CAD build for the part. Positions are in the model's coordinates, mm. Face numbers are marked on the shaded views. A direction names the side the tool comes from. Give positions to 0.01 mm unless a question says otherwise; leave off trailing zeros. Write each loop counter-clockwise with the first axis right and the second up, starting at its lowest first coordinate (ties: lowest second). Pieces come first, ordered by that corner, then holes. Notation, with made-up numbers: (50, 38.5) -> (109, 38.5) arc R9 ccw to (109, 53.5) -> close; hole circle Ø2 at (12.5, 20.25). An arc over 180 degrees is marked (long way). Use one line per item in the form item = value. Start each with the question number.
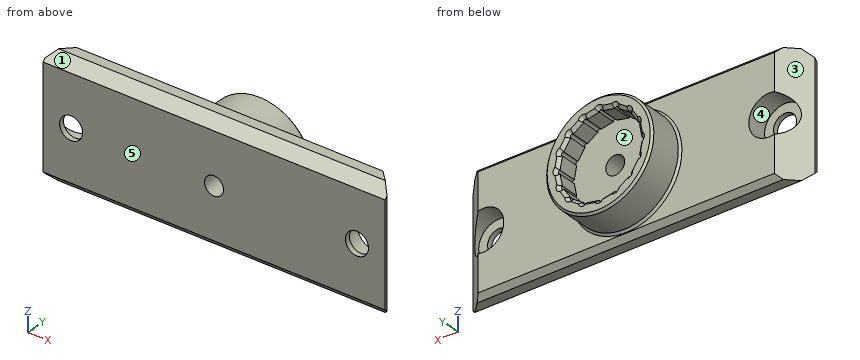
from build123d import *

# Parameters (mm, degrees)
SKETCH1_W                      = 67
SKETCH1_H                      = 24
BOSS_EXTRUDE1_DEPTH            = 5
SKETCH2_R                      = 10.5
BOSS_EXTRUDE2_DEPTH            = 7
CBORE_START                    = 1
CBORE_FOR_M4_SHCS1_OUTLINE_R   = 4
CBORE_FOR_M4_SHCS1_DEPTH       = 4
CBORE_FOR_M4_SHCS1_2_OUTLINE_R = 2.25
CBORE_FOR_M4_SHCS1_2_DEPTH     = 1
CHAMFER1_SIZE                  = 1
CHAMFER2_SIZE                  = 2
SKETCH5_OUTSIDE_W              = 83.434
SKETCH5_OUTSIDE_H              = 28.434
CUT_EXTRUDE1_DEPTH             = 43.921439864
SKETCH6_R                      = 10.5
BOSS_EXTRUDE3_DEPTH            = 7
CHAMFER4_SIZE                  = 0.4
HOLE1_D                        = 3.7
HOLE1_DEPTH                    = 16
HOLE1_TIP                      = 1.85
CUT_EXTRUDE2_DEPTH             = 4.2
SKETCH12_R                     = 0.35
CUT_EXTRUDE3_DEPTH             = 4.2
CHAMFER5_SIZE                  = 0.6


# Read off the part's stored shape, not the designer's step: CBORE for M4 SHCS1
with BuildPart() as part:
    # Sketch1 → Boss-Extrude1 (new body)
    with BuildSketch(Plane(origin=(0, 0, 0), x_dir=(1, 0, 0), z_dir=(0, 1, 0))):
        Rectangle(SKETCH1_W, SKETCH1_H)
    extrude(amount=BOSS_EXTRUDE1_DEPTH)

    # Sketch2 → Boss-Extrude2 (add)
    with BuildSketch(Plane(origin=(0, 5, 0), x_dir=(1, 0, 0), z_dir=(0, 1, 0))):
        with Locations(Location((0, 0, 0), (0, 0, 270))):
            Circle(SKETCH2_R)
    extrude(amount=BOSS_EXTRUDE2_DEPTH)

    # CBORE for M4 SHCS1 outline → CBORE for M4 SHCS1 (cut)
    with BuildSketch(Plane(origin=(0, 0, 0), x_dir=(1, 0, 0), z_dir=(0, 1, 0)).offset(CBORE_START)):
        with Locations((28, 0)):
            Circle(CBORE_FOR_M4_SHCS1_OUTLINE_R)
        with Locations((-28, 0)):
            Circle(CBORE_FOR_M4_SHCS1_OUTLINE_R)
    extrude(amount=CBORE_FOR_M4_SHCS1_DEPTH, mode=Mode.SUBTRACT)

    # CBORE for M4 SHCS1 2 outline → CBORE for M4 SHCS1 2 (cut)
    with BuildSketch(Plane(origin=(0, 0, 0), x_dir=(1, 0, 0), z_dir=(0, 1, 0))):
        with Locations((28, 0)):
            Circle(CBORE_FOR_M4_SHCS1_2_OUTLINE_R)
        with Locations((-28, 0)):
            Circle(CBORE_FOR_M4_SHCS1_2_OUTLINE_R)
    extrude(amount=CBORE_FOR_M4_SHCS1_2_DEPTH, mode=Mode.SUBTRACT)

    # Chamfer1
    chamfer1_edges = [part.edges().sort_by_distance(p)[0] for p in [
        (-33.5, 5, 0),
        (0, 5, 12),
        (33.5, 5, 0),
        (33.5, 2.5, 12),
        (-33.5, 2.5, 12),
        (-33.5, 2.5, -12),
        (33.5, 2.5, -12),
        (0, 5, -12),
    ]]
    chamfer(chamfer1_edges, length=CHAMFER1_SIZE)

    # Chamfer2
    chamfer2_edges = [part.edges().sort_by_distance(p)[0] for p in [
        (0, 0, -12),
        (0, 0, 12),
    ]]
    chamfer(chamfer2_edges, length=CHAMFER2_SIZE)

    # Sketch5 outside → Cut-Extrude1 (cut, through all)
    with BuildSketch(Plane.XY.offset(12)):
        with Locations((0, 6)):
            Rectangle(SKETCH5_OUTSIDE_W, SKETCH5_OUTSIDE_H)
        Polygon((-34, 0), (-22, 12), (22, 12), (34, 0), align=None, mode=Mode.SUBTRACT)
    extrude(amount=-CUT_EXTRUDE1_DEPTH, mode=Mode.SUBTRACT)

    # Sketch6 → Boss-Extrude3 (add)
    with BuildSketch(Plane(origin=(0, 5, 0), x_dir=(1, 0, 0), z_dir=(0, 1, 0))):
        with Locations(Location((0, 0, 0), (0, 0, 270))):
            Circle(SKETCH6_R)
    extrude(amount=BOSS_EXTRUDE3_DEPTH)

    # Chamfer4
    chamfer4_edges = [part.edges().sort_by_distance(p)[0] for p in [
        (0, 5, -10.5),
        (0, 12, -10.5),
    ]]
    chamfer(chamfer4_edges, length=CHAMFER4_SIZE)

    # Hole1
    with Locations(Plane(origin=(0, 12, 0), x_dir=(1, 0, 0), z_dir=(0, 1, 0))):
        with Locations((0, 0)):
            Hole(HOLE1_D / 2, depth=HOLE1_DEPTH)
            with Locations((0, 0, -(HOLE1_DEPTH + HOLE1_TIP / 2))):  # 90° drill point
                Cone(0, HOLE1_D / 2, HOLE1_TIP, mode=Mode.SUBTRACT)

    # Sketch11 → Cut-Extrude2 (cut)
    with BuildSketch(Plane(origin=(0, 12, 0), x_dir=(1, 0, 0), z_dir=(0, 1, 0))):
        Polygon((0, 8.1), (-3.099735802, 7.483424213), (-5.727564928, 5.727564928), (-7.483424213, 3.099735802), (-8.1, 0), (-7.483424213, -3.099735802), (-5.727564928, -5.727564928), (-3.099735802, -7.483424213), (0, -8.1), (3.099735802, -7.483424213), (5.727564928, -5.727564928), (7.483424213, -3.099735802), (8.1, 0), (7.483424213, 3.099735802), (5.727564928, 5.727564928), (3.099735802, 7.483424213), align=None)
    extrude(amount=-CUT_EXTRUDE2_DEPTH, mode=Mode.SUBTRACT)

    # Sketch12 → Cut-Extrude3 (cut)
    with BuildSketch(Plane(origin=(0, 12, 0), x_dir=(1, 0, 0), z_dir=(0, 1, 0))):
        with Locations((0, 8)):
            Circle(SKETCH12_R)
        with Locations((3.061467459, 7.39103626)):
            Circle(SKETCH12_R)
        with Locations((5.656854249, 5.656854249)):
            Circle(SKETCH12_R)
        with Locations((7.39103626, 3.061467459)):
            Circle(SKETCH12_R)
        with Locations((8, 0)):
            Circle(SKETCH12_R)
        with Locations((7.39103626, -3.061467459)):
            Circle(SKETCH12_R)
        with Locations((5.656854249, -5.656854249)):
            Circle(SKETCH12_R)
        with Locations((3.061467459, -7.39103626)):
            Circle(SKETCH12_R)
        with Locations((0, -8)):
            Circle(SKETCH12_R)
        with Locations((-3.061467459, -7.39103626)):
            Circle(SKETCH12_R)
        with Locations((-5.656854249, -5.656854249)):
            Circle(SKETCH12_R)
        with Locations((-7.39103626, -3.061467459)):
            Circle(SKETCH12_R)
        with Locations((-8, 0)):
            Circle(SKETCH12_R)
        with Locations((-7.39103626, 3.061467459)):
            Circle(SKETCH12_R)
        with Locations((-5.656854249, 5.656854249)):
            Circle(SKETCH12_R)
        with Locations((-3.061467459, 7.39103626)):
            Circle(SKETCH12_R)
    extrude(amount=-CUT_EXTRUDE3_DEPTH, mode=Mode.SUBTRACT)

    # Chamfer5
    chamfer5_edges = [part.edges().sort_by_distance(p)[0] for p in [
        (-1.549867901, 12, -7.791712107),
        (-4.413650365, 12, -6.60549457),
        (-6.60549457, 12, -4.413650365),
        (-7.791712107, 12, -1.549867901),
        (-7.791712107, 12, 1.549867901),
        (-6.60549457, 12, 4.413650365),
        (-4.413650365, 12, 6.60549457),
        (-1.549867901, 12, 7.791712107),
        (1.549867901, 12, 7.791712107),
        (4.413650365, 12, 6.60549457),
        (6.60549457, 12, 4.413650365),
        (7.791712107, 12, 1.549867901),
        (7.791712107, 12, -1.549867901),
        (6.60549457, 12, -4.413650365),
        (4.413650365, 12, -6.60549457),
        (1.549867901, 12, -7.791712107),
        (-3.19540666, 12, -7.714394096),
        (-5.904341623, 12, -5.904341623),
        (-7.714394096, 12, -3.19540666),
        (-8.35, 12, 0),
        (-7.714394096, 12, 3.19540666),
        (-5.904341623, 12, 5.904341623),
        (-3.19540666, 12, 7.714394096),
        (0, 12, 8.35),
        (3.19540666, 12, 7.714394096),
        (5.904341623, 12, 5.904341623),
        (7.714394096, 12, 3.19540666),
        (8.35, 12, 0),
        (7.714394096, 12, -3.19540666),
        (5.904341623, 12, -5.904341623),
        (3.19540666, 12, -7.714394096),
        (0, 12, -8.35),
    ]]
    chamfer(chamfer5_edges, length=CHAMFER5_SIZE)


solid = part.part
1) Cut at C-C (x = -28). Give the cut face in (y, z), and give its area (3 significant figures).
2) 3-axis set-ups, long thin cutter, end or side, ignore diameter. For the marked faces 4 and 5: which of +Z, -Z, +X, -X, +Y, -Y reach the whole face in a straight line?
3) Wall check: line 1 along Z through (x, y) = (-30, 2); line 2 along Y through (x, z) = (-22.5, 7.25); line 3 along Z through (x, y) = (-16, 0.5). Give the ranges that are in metal, low to high. Write a range as from..to.
4) Two-plate mould, pull along Z, no slides. Class the marked faces 1, 2 and 3: released by +Z, released by -Z, zero draft, split by the parting line, or undercut.
5) Cut at B-B (x = -17). Give the cut face in (y, z).
6) Cut at D-D (y = 3). Give the cut face in (x, z).
7) Pin check, flat tips, straight feed: pin 1 (7 mm diameter, centred on x = 28, z = 0, fed in from +Y); pin 2 (4 mm diameter, centred on x = -28, z = 0, fed in from +Y); pin 3 (11 mm diameter, centred on x = 0, z = -2, fed in from +Y); pin 4 (9 mm diameter, centred on x = -27, z = -1, fed in from +Y). Stop position of each tip, or through.
Final values:
q1.outline = (0, -10) -> (2, -12) -> (4, -12) -> (5, -11) -> (5, -4) -> (1, -4) -> (1, -2.25) -> (0, -2.25) -> close; (0, 2.25) -> (1, 2.25) -> (1, 4) -> (5, 4) -> (5, 11) -> (4, 12) -> (2, 12) -> (0, 10) -> close
q1.area = 78.5 mm^2
q2.face_4 = +Y
q2.face_5 = +Z, -Z, +X, -X, -Y
q3.line_1 = -12..-3.46, 3.46..12
q3.line_2 = 0..5
q3.line_3 = -10.5..10.5
q4.face_1 = released by +Z
q4.face_2 = undercut
q4.face_3 = zero draft
q5.outline = (0, -10) -> (2, -12) -> (4, -12) -> (5, -11) -> (5, 11) -> (4, 12) -> (2, 12) -> (0, 10) -> close
q6.outline = (-31, -12) -> (31, -12) -> (31, -2.65) arc R4 cw (long way) to (31, 2.65) -> (31, 12) -> (-31, 12) -> (-31, 2.65) arc R4 cw (long way) to (-31, -2.65) -> close; hole circle Ø3.7 at (0, 0)
q7.pin_1 = 1
q7.pin_2 = through
q7.pin_3 = 7.8
q7.pin_4 = 5
